Here's how the part is built. I have some questions about the finished solid (model axes, mm). A direction names the side the tool comes from. Round coordinates to 2 decimals unless told otherwise and drop trailing zeros. Order: outer loops, then holes, each group sorted by start corner. A loop starts at its lowest first (then second) coordinate and runs counter-clockwise, first axis right, second up.
```python
from build123d import *
from build123d.topology import SkipClean

# Parameters (mm, degrees)
CROQUIS1_W              = 38.578820375
CROQUIS1_H              = 46.492266094
SALIENTE_EXTRUIR1_DEPTH = 36
CROQUIS2_R              = 13.723036729
CORTAR_EXTRUIR1_DEPTH   = 54
REDONDEO1_R             = 35
SALIENTE_EXTRUIR2_DEPTH = 16
CROQUIS4_R              = 13.723036729
CORTAR_EXTRUIR2_DEPTH   = 14
CROQUIS5_W              = 15.936830691
CROQUIS5_H              = 4.692990875
CORTAR_EXTRUIR3_DEPTH   = 54
CROQUIS6_W              = 15.323001746
CROQUIS6_H              = 19.007540334
CORTAR_EXTRUIR4_DEPTH   = 54


with BuildPart() as part:
    # Croquis1 → Saliente-Extruir1 (new body)
    with BuildSketch(Plane.XY):
        with Locations((-55.636003999, -7.514612749)):
            Rectangle(CROQUIS1_W, CROQUIS1_H)
    extrude(amount=SALIENTE_EXTRUIR1_DEPTH)

    # Croquis2 → Cortar-Extruir1 (cut)
    with BuildSketch(Plane.ZY.offset(74.925414186)):
        with Locations((15.035056118, -8.31763911)):
            Circle(CROQUIS2_R)
    extrude(amount=-CORTAR_EXTRUIR1_DEPTH, mode=Mode.SUBTRACT)

    # Redondeo1
    # the kernel refuses this fillet: 35 mm, written as the material it takes off along each edge
    with BuildSketch(Plane(origin=(51.153406189, 15.731520298, 36), x_dir=(0, 0, -1), z_dir=(-1, 0, 0))) as redondeo1_piece_1:
        with BuildLine():
            CenterArc((REDONDEO1_R, REDONDEO1_R), REDONDEO1_R, 180, 90)
            Line((0, REDONDEO1_R), (0, 0))
            Line((0, 0), (REDONDEO1_R, 0))
        make_face()
    extrude(amount=213.578820376, mode=Mode.SUBTRACT)
    with BuildSketch(Plane(origin=(-162.425414186, -30.760745796, 36), x_dir=(0, 1, 0), z_dir=(1, 0, 0))) as redondeo1_piece_2:
        with BuildLine():
            CenterArc((REDONDEO1_R, -REDONDEO1_R), REDONDEO1_R, 90, 90)
            Line((0, -REDONDEO1_R), (0, 0))
            Line((0, 0), (REDONDEO1_R, 0))
        make_face()
    extrude(amount=213.578820376, mode=Mode.SUBTRACT)

    # Croquis3 → Saliente-Extruir2 (add)
    with BuildSketch(Plane(origin=(-36.346593811, 0, 0), x_dir=(0, 0, -1), z_dir=(1, 0, 0))):
        with BuildLine():
            Line((0, 15.731520298), (-1, 15.731520298))
            ThreePointArc((-1, 15.731520298), (-21.169465246, 9.335587695), (-33.967356759, -7.514612749))
            ThreePointArc((-33.967356759, -7.514612749), (-21.169465246, -24.364813193), (-1, -30.760745796))
            Line((-1, -30.760745796), (0, -30.760745796))
            Line((0, -30.760745796), (0, 15.731520298))
        make_face()
    extrude(amount=SALIENTE_EXTRUIR2_DEPTH)

    # Croquis4 → Cortar-Extruir2 (cut)
    with SkipClean():  # the faces are left unmerged after this step: merging them gives an invalid solid
        with BuildSketch(Plane.ZY.offset(36.346593811)):
            with Locations((15.035056118, -8.31763911)):
                Circle(CROQUIS4_R)
        extrude(amount=-CORTAR_EXTRUIR2_DEPTH, mode=Mode.SUBTRACT)

    # Croquis5 → Cortar-Extruir3 (cut)
    with SkipClean():  # the faces are left unmerged after this step: merging them gives an invalid solid
        with BuildSketch(Plane.ZY.offset(74.925414186)):
            with Locations((14.642217913, 4.910546276)):
                Rectangle(CROQUIS5_W, CROQUIS5_H)
        extrude(amount=-CORTAR_EXTRUIR3_DEPTH, mode=Mode.SUBTRACT)

    # Croquis6 → Cortar-Extruir4 (cut)
    with SkipClean():  # the faces are left unmerged after this step: merging them gives an invalid solid
        with BuildSketch(Plane.XZ.offset(-7.257041714)):
            with Locations((-28.598941082, 16.267176719)):
                Rectangle(CROQUIS6_W, CROQUIS6_H)
        extrude(amount=-CORTAR_EXTRUIR4_DEPTH, mode=Mode.SUBTRACT)


solid = part.part
```
1. I'm going to push flat-ended pins straight in: P1, Ø4, axis at x = -44, z = 21.5, coming from the -Y side; P2, Ø4, axis at x = -38, y = 6, coming from the +Z side; P3, Ø1, axis at x = -31.5, z = 23, coming from the +Y side. Where does each tip first touch, or does it pass through?
Evaluation:
P1: stops at y = -25.47
P2: stops at z = 27.15
P3: stops at y = 7.26
2. If we section it at A-A, the plane x = -65.5: Write out the boundary of the cut face in (y, z).
Evaluation:
outline: (-30.76, 0) - (15.73, 0) - (15.73, 1) arc R35 ccw to (-7.51, 33.97) arc R35 ccw to (-30.76, 1) - close; hole (2.56, 6.67) - (7.26, 6.67) - (7.26, 22.61) - (3.12, 22.61) arc R13.72 ccw (long way) to start
3. If we section it at C-C, the plane x = -25: Write out the boundary of the cut face in (y, z), and give its area (3 significant figures).
Evaluation:
outline: (-30.76, 0) - (15.73, 0) - (15.73, 1) arc R35 ccw to (15.25, 6.76) - (7.26, 6.76) - (7.26, 6.67) - (2.56, 6.67) arc R13.72 cw (long way) to (3.12, 22.61) - (7.26, 22.61) - (7.26, 23.83) arc R35 ccw to (-7.51, 33.97) arc R35 ccw to (-30.76, 1) - close
area: 445 mm2
4. If we section it at D-D, the plane y = -13: Write out the boundary of the cut face in (x, z).
Evaluation:
outline: (-74.93, 0) - (-20.35, 0) - (-20.35, 31.46) - (-74.93, 31.46) - (-74.93, 27.93) - (-22.35, 27.93) - (-22.35, 2.14) - (-74.93, 2.14) - close
5. I need wall thicknesses on probe 1 along X at (y, z) = (-14, 5.5); probe 2 along Z at (x, y) = (-51, -3.5); probe 3 along Y at (x, z) = (-48, 25.5). Which ranges of each line are inside material? Lowest first, please.
Evaluation:
probe 1: x = -22.35 to -20.35
probe 2: z = 0 to 2.19, 27.88 to 32.25
probe 3: y = -20.76 to -17.19, 0.56 to 5.73
6. If we mould it in two halves opening along X, with no side actions, what happens to faces 1 (the flat face through (-29, 7.257, 23)), 2 (the flat face through (-54, 7.257, 15)), 3 (the flat face through (-22.347, -9, 15))? For each: released by +X, released by -X, zero draft, split by the parting line, or undercut.
Evaluation:
face 1: undercut
face 2: zero draft
face 3: released by -X
7. On a 3-axis mill with a long thin cutter (end or side, diameter ignored), from which of +Z, -Z, +X, -X, +Y, -Y can I reach the whole of each face in a straight line? I mean faces 4 (the flat face through (-48, 5, 22.611)), 5 (the flat face through (-20.347, -7, 13)), 6 (the flat face through (-29, 11, 6.763)). Say none if no direction works.
Evaluation:
face 4: -X
face 5: +Z, -Z, +X, +Y, -Y
face 6: +Z, +Y
